Job drawing, mm, ordinate dimensions from the low corner. One solid piece. A direction names the side the tool comes from. Coordinates: 2 decimals unless noted, no trailing zeros. Write each loop counter-clockwise with the first axis right and the second up, starting at its lowest first coordinate (ties: lowest second). Pieces come first, ordered by that corner, then holes.
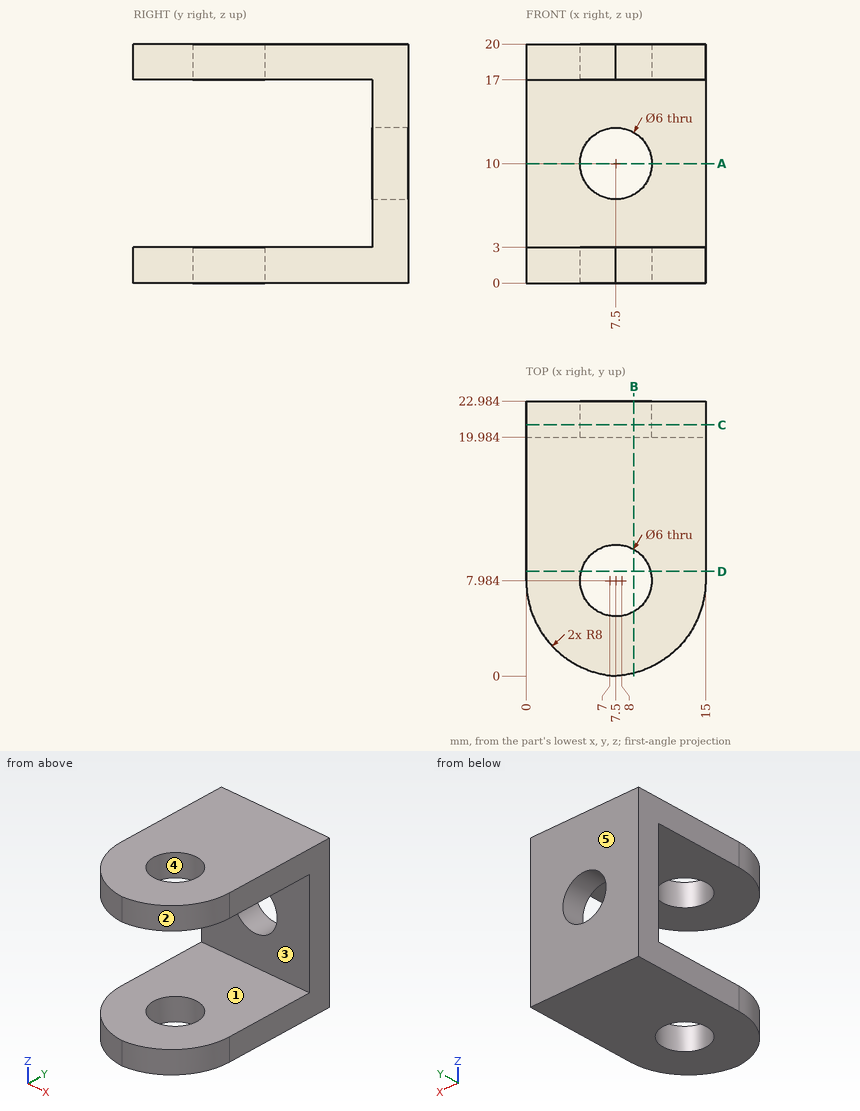
1. Probe line 1 along Z through (x, y) = (5, 12.25); line 2 along Y through (x, z) = (7.5, 17.8) (1 decimal); line 3 along X through (y, z) = (20.8, 10). List the from-to ranges inside material, lowest first.
Computed values:
line 1: z = 0 to 3, 17 to 20
line 2: y = 0 to 5, 11 to 23
line 3: x = 0 to 4.5, 10.5 to 15
2. Flat gauge pins, fed straight in: pin 1 (7 mm diameter, centred on x = 7.5, y = 7.98, fed in from +Z); pin 2 (8 mm diameter, centred on x = 7.5, z = 10, fed in from -Y). Where does each tip first touch, or does it go through?
Computed values:
pin 1: stops at z = 20
pin 2: stops at y = 19.98
3. 3-axis set-ups, long thin cutter, end or side, ignore diameter. For the marked faces 1 and 2: which of +Z, -Z, +X, -X, +Y, -Y reach the whole face in a straight line?
Computed values:
face 1: +X, -X, -Y
face 2: +Z, -Z, +X, -Y
4. Mould opens along Y. For the marked faces 3, 4 and 5 say: +Y half, -Y half, draft (parallel to the pull), parting line (faces both ways), or undercut.
Computed values:
face 3: -Y half
face 4: undercut
face 5: +Y half
5. Saw through at B-B on x = 9. List the corners of the cut face in (y, z) (1 decimal), plus the area to 3 significant figures.
Computed values:
outline: (0.2, 0) - (5.4, 0) - (5.4, 3) - (0.2, 3) - close; (0.2, 17) - (5.4, 17) - (5.4, 20) - (0.2, 20) - close; (10.6, 0) - (23, 0) - (23, 7.4) - (20, 7.4) - (20, 3) - (10.6, 3) - close; (10.6, 17) - (20, 17) - (20, 12.6) - (23, 12.6) - (23, 20) - (10.6, 20) - close
area: 132 mm2
6. Saw through at C-C on y = 21. List the corners of the cut face in (x, z), plus the area to 3 significant figures.
Computed values:
outline: (0, 0) - (15, 0) - (15, 20) - (0, 20) - close; hole circle Ø6 at (7.5, 10)
area: 272 mm2
7. Saw through at D-D on y = 8.75. List the corners of the cut face in (x, z).
Computed values:
outline: (0, 0) - (4.6, 0) - (4.6, 3) - (0, 3) - close; (0, 17) - (4.6, 17) - (4.6, 20) - (0, 20) - close; (10.4, 0) - (15, 0) - (15, 3) - (10.4, 3) - close; (10.4, 17) - (15, 17) - (15, 20) - (10.4, 20) - close
8. Saw through at A-A on z = 10. List the corners of the cut face in (x, y) (1 decimal).
Computed values:
outline: (0, 20) - (4.5, 20) - (4.5, 23) - (0, 23) - close; (10.5, 20) - (15, 20) - (15, 23) - (10.5, 23) - close
